Design review of the part built by this model. Coordinates are the model's own, in mm. A direction names the side the tool comes from. Give positions to 0.01 mm unless a question says otherwise; leave off trailing zeros. Loops run counter-clockwise (first coordinate to the right, second up) from the corner with the lowest first, then second, coordinate; pieces in that order, holes last. Notation, with made-up numbers: (62, 71) -> (107, 71) arc R18 ccw to (107, 85) -> close; hole circle Ø11 at (-3, 42.5). An arc over 180 degrees is marked (long way). Answer as CSV lines item,"result".
from build123d import *

# Parameters (mm, degrees)
SKETCH1_R           = 10
SKETCH1_R_2         = 7.5
BOSS_EXTRUDE1_DEPTH = 10
SKETCH6_R           = 10
BOSS_EXTRUDE3_DEPTH = 20
BOSS_EXTRUDE3_TAPER = -60
SKETCH8_R           = 7.5
CUT_EXTRUDE3_DEPTH  = 20
CUT_EXTRUDE3_TAPER  = -58


with BuildPart() as part:
    # Sketch1 → Boss-Extrude1 (new body)
    with BuildSketch(Plane(origin=(0, 0, 0), x_dir=(1, 0, 0), z_dir=(0, 1, 0))):
        Circle(SKETCH1_R)
        Circle(SKETCH1_R_2, mode=Mode.SUBTRACT)
    extrude(amount=BOSS_EXTRUDE1_DEPTH)

    # Sketch6 → Boss-Extrude3 (add)
    with BuildSketch(Plane(origin=(0, 10, 0), x_dir=(1, 0, 0), z_dir=(0, 1, 0))):
        Circle(SKETCH6_R)
    extrude(amount=BOSS_EXTRUDE3_DEPTH, taper=BOSS_EXTRUDE3_TAPER)

    # Sketch8 → Cut-Extrude3 (cut)
    with BuildSketch(Plane.XZ.offset(-10)):
        Circle(SKETCH8_R)
    extrude(amount=-CUT_EXTRUDE3_DEPTH, taper=CUT_EXTRUDE3_TAPER, mode=Mode.SUBTRACT)


solid = part.part
Q1. We need section C-C, the plane y = 17. State the section outline as (x, z) points.
Filled sheet:
outline,"circle Ø44.25 at (0, 0); hole circle Ø37.4 at (0, 0)"
Q2. We need section B-B, the plane y = 6.5. State the section outline as (x, z) points.
Filled sheet:
outline,"circle Ø20 at (0, 0); hole circle Ø15 at (0, 0)"
Q3. For faces 1 (the cylindrical face through (-7.493, 4.93, -0.33)), 2 (the cylindrical face through (-2.17, 4.93, 9.76)), list the 3-axis set-ups (+Z, -Z, +X, -X, +Y, -Y) from which the entire face can be reached by the end or side of a thin tool; tool diameter is ignored.
Filled sheet:
face 1,"+Y, -Y"
face 2,"-Y"
Q4. Clearance check with flat-ended pins moving along their axes: pin 1 Ø6 at (x, y) = (-18.5, 25) entering from +Z; pin 2 Ø6 at (x, z) = (25, 34) entering from -Y; pin 3 Ø1.5 at (y, z) = (5, -2.5) entering from +X; pin 4 Ø24 at (x, z) = (0, 0) entering from -Y. State where each tip first meets the part, or that it passes through.
Filled sheet:
pin 1,"stops at z = 36.97"
pin 2,"stops at y = 26.86"
pin 3,"stops at x = 9.85"
pin 4,"stops at y = 0"
Q5. To check wall thickness, follow probe 1 along X at (y, z) = (4, 0); probe 2 along Z at (x, y) = (-24.5, 25.5). State the ranges of each line that lie inside material, in increasing order. Write a range as from..to.
Filled sheet:
probe 1,"x = -10..-7.5, 7.5..10"
probe 2,"z = -27.52..-21.06, 21.06..27.52"
Q6. We need section A-A, the plane x = 0. State the section outline as (y, z) points, and give its area (3 significant figures).
Filled sheet:
outline,"(0, -10) -> (10, -10) -> (30, -44.64) -> (30, -39.51) -> (10, -7.5) -> (0, -7.5) -> close; (0, 7.5) -> (10, 7.5) -> (30, 39.51) -> (30, 44.64) -> (10, 10) -> (0, 10) -> close"
area,"203 mm^2"
